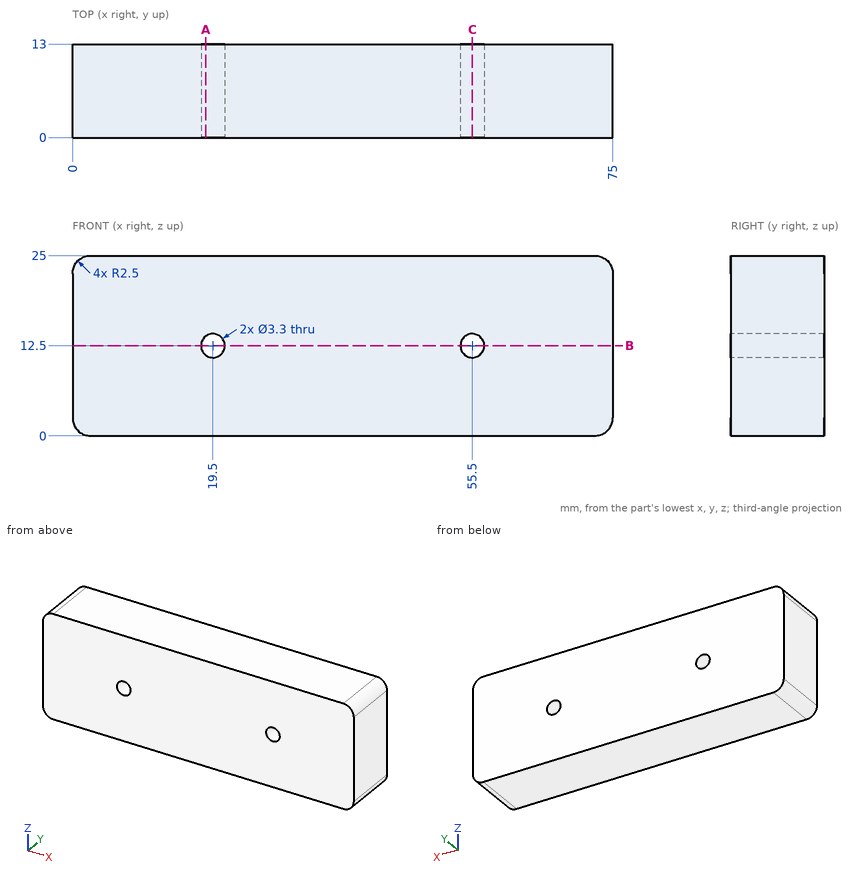
Study the drawing (mm; zero at the part's minimum x, y, z) and answer. Give positions to 0.01 mm unless a question says otherwise; leave off trailing zeros. Loops run counter-clockwise (first coordinate to the right, second up) from the corner with the lowest first, then second, coordinate; pieces in that order, holes last. Notation, with made-up numbers: (0.5, 29.25) -> (49.5, 29.25) arc R31 ccw to (49.5, 66.25) -> close; hole circle Ø6 at (57, -10). An arc over 180 degrees is marked (long way). Write item = value, one per line. Start each with the question number.
(1) Find section C-C on x = 55.5. Give the vertices of the cut face in (y, z), and give its area (3 significant figures).
(2) Find the intervals of material crossed by probe 1 along X at (y, z) = (4.25, 12.5); probe 2 along Z at (x, y) = (55.5, 7.75); probe 3 along X at (y, z) = (10.5, 23.25), in increasing order. Write a range as from..to.
(3) Given pin 1 Ø3 at (x, z) = (19.5, 12.5) entering from +Y, flat-ended and moving along its own axis, determine where the tip first touches the part or whether it passes through.
(4) Find section B-B on z = 12.5. Give the vertices of the cut face in (x, y), and give its area (3 significant figures).
(5) Find section A-A on x = 18.5. Give the vertices of the cut face in (y, z), and give its area (3 significant figures).
From the geometry:
q1.outline = (0, 0) -> (13, 0) -> (13, 10.85) -> (0, 10.85) -> close; (0, 14.15) -> (13, 14.15) -> (13, 25) -> (0, 25) -> close
q1.area = 282 mm^2
q2.probe_1 = 0..17.85, 21.15..53.85, 57.15..75
q2.probe_2 = 0..10.85, 14.15..25
q2.probe_3 = 0.12..74.88
q3.pin_1 = through
q4.outline = (0, 0) -> (17.85, 0) -> (17.85, 13) -> (0, 13) -> close; (21.15, 0) -> (53.85, 0) -> (53.85, 13) -> (21.15, 13) -> close; (57.15, 0) -> (75, 0) -> (75, 13) -> (57.15, 13) -> close
q4.area = 889 mm^2
q5.outline = (0, 0) -> (13, 0) -> (13, 11.19) -> (0, 11.19) -> close; (0, 13.81) -> (13, 13.81) -> (13, 25) -> (0, 25) -> close
q5.area = 291 mm^2
